```python
from build123d import *

# Parameters (mm, degrees)
SKETCH1_W           = 7
SKETCH1_H           = 65
SKETCH1_R           = 2.5
SKETCH1_H_2         = 33
BOSS_EXTRUDE1_DEPTH = 22.325
SKETCH2_R           = 17.825
CUT_EXTRUDE1_DEPTH  = 74.305222358
SKETCH3_R           = 6
CUT_EXTRUDE2_DEPTH  = 22.325


with BuildPart() as part:
    # Sketch1 → Boss-Extrude1 (new body)
    # profile 1 of 3: a face of its own
    with BuildSketch(Plane(origin=(0, 0, 0), x_dir=(1, 0, 0), z_dir=(0, 1, 0))):
        with Locations((22, 0)):
            Rectangle(SKETCH1_W, SKETCH1_H)
        with Locations(Location((22, -16.25, 0), (0, 0, 90))):
            Circle(SKETCH1_R, mode=Mode.SUBTRACT)
        with Locations(Location((22, 16.25, 0), (0, 0, 90))):
            Circle(SKETCH1_R, mode=Mode.SUBTRACT)
    # profile 2 of 3: a face of its own
    with BuildSketch(Plane(origin=(0, 0, 0), x_dir=(1, 0, 0), z_dir=(0, 1, 0))):
        with BuildLine():
            Line((-18.5, 32.5), (-18.5, -0.5))
            ThreePointArc((-18.5, -0.5), (-6.523379041, -14.840809158), (-0.42, -32.5))
            Line((-0.42, -32.5), (18.5, -32.5))
            Line((18.5, -32.5), (18.5, 32.5))
            Line((18.5, 32.5), (-18.5, 32.5))
        make_face()
    # profile 3 of 3: a face of its own
    with BuildSketch(Plane(origin=(0, 0, 0), x_dir=(1, 0, 0), z_dir=(0, 1, 0))):
        with Locations((-22, 16)):
            Rectangle(SKETCH1_W, SKETCH1_H_2)
        with Locations(Location((-22, 7.5, 0), (0, 0, 90))):
            Circle(SKETCH1_R, mode=Mode.SUBTRACT)
        with Locations(Location((-22, 24.5, 0), (0, 0, 90))):
            Circle(SKETCH1_R, mode=Mode.SUBTRACT)
    extrude(amount=BOSS_EXTRUDE1_DEPTH)

    # Sketch2 → Cut-Extrude1 (cut, through all)
    with BuildSketch(Plane(origin=(0, 0, -32.5), x_dir=(-1, 0, 0), z_dir=(0, 0, -1))):
        with Locations((0, 22.325)):
            Circle(SKETCH2_R)
        with BuildLine():
            Line((-17.825, 8.88345991), (-25.5, 8.88345991))
            Line((-25.5, 8.88345991), (-25.5, -2.88343075))
            Line((-25.5, -2.88343075), (25.5, -2.88343075))
            Line((25.5, -2.88343075), (25.5, 8.88345991))
            Line((25.5, 8.88345991), (17.825, 8.88345991))
            ThreePointArc((17.825, 8.88345991), (0, 0), (-17.825, 8.88345991))
        make_face()
    extrude(amount=-CUT_EXTRUDE1_DEPTH, mode=Mode.SUBTRACT)

    # Sketch3 → Cut-Extrude2 (cut)
    with BuildSketch(Plane.XZ.offset(-8.88345991)):
        with Locations((-22, -7.5)):
            Circle(SKETCH3_R)
        with Locations((22, -16.25)):
            Circle(SKETCH3_R)
        with Locations((22, 16.25)):
            Circle(SKETCH3_R)
        with Locations((-22, -24.5)):
            Circle(SKETCH3_R)
    extrude(amount=CUT_EXTRUDE2_DEPTH, mode=Mode.SUBTRACT)


with BuildPart() as body_2:
    # Mirror2: mirrored copy
    add(part.part.mirror(Plane(origin=(-25.5, 22.325, 0), x_dir=(0, 0, 1), z_dir=(-1, 0, 0))))


solid = body_2.part
```
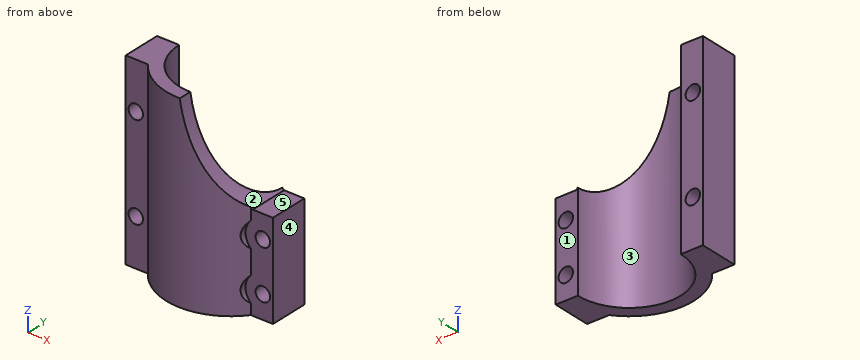
Model file for the job. Use its own axes, mm. Face numbers are marked on the shaded views. A direction names the side the tool comes from. Coordinates: 2 decimals unless noted, no trailing zeros. Order: outer loops, then holes, each group sorted by start corner. A loop starts at its lowest first (then second) coordinate and runs counter-clockwise, first axis right, second up. Notation, with made-up numbers: (31, 73) - (48, 73) arc R4 ccw to (48, 78) - close; hole circle Ø2 at (67, -38.5). An arc over 180 degrees is marked (long way). Return JSON: item names as keys, results as strings. Group by question number.
1) Mould opens along X. For the marked faces 1, 2 and 3 say: released by +X, released by -X, zero draft, split by the parting line, or undercut.
2) Saw through at A-A, the plane z = -7.5. Write the cut outline in (x, y) (3 decimals), plus the area to 3 significant figures.
3) Saw through at B-B, the plane y = 14. Write the cut outline in (x, z).
4) Saw through at C-C, the plane y = 20. Write the cut outline in (x, z), plus the area to 3 significant figures.
5) Flat gauge pins, fed straight in: P1, Ø8, axis at x = -39.5, z = 5.5, coming from the -Y side; P2, Ø10.5, axis at x = -28, z = -15, coming from the -Y side; P3, Ø5, axis at y = 10, z = 9.5, coming from the +X side; P4, Ø4.5, axis at x = -73, z = 16.25, coming from the -Y side. Where does each tip first touch, or does it go through?
6) Tool access for the marked faces 4 and 5: list every direction of +Z, -Z, +X, -X, +Y, -Y with a clear straight run to the whole face (end or side of a thin tool).
7) Saw through at D-D, the plane x = -34. Write the cut outline in (y, z), plus the area to 3 significant figures.
8) Probe line 1 (Z direction, x = -29, y = 17.75); line 2 (X direction, y = 17.75, z = -24.5); line 3 (X direction, y = 17.75, z = -6). List the from-to ranges inside material, lowest first. Write a range as from..to.
Values found:
{
 "1": {"face 1": "zero draft", "face 2": "released by +X", "face 3": "undercut"},
 "2": {"outline": "(-76.5, 8.883) - (-68.825, 8.883) arc R22.325 ccw to (-35, 6.756) - (-35, 8.883) - (-31.5, 8.883) - (-31.5, 22.325) - (-33.175, 22.325) arc R17.825 cw to (-68.825, 22.325) - (-76.5, 22.325) - close; (-26.5, 8.883) - (-25.5, 8.883) - (-25.5, 22.325) - (-26.5, 22.325) - close", "area": "338 mm²"},
 "3": {"outline": "(-76.5, -32.5) - (-66.76, -32.5) - (-66.76, 32.5) - (-76.5, 32.5) - close; (-35.24, -32.5) - (-25.5, -32.5) - (-25.5, 0.5) - (-32.5, 0.5) arc R51.75 cw to (-35.24, 2.95) - close; hole circle Ø5 at (-73, -16.25); hole circle Ø5 at (-73, 16.25); hole circle Ø5 at (-29, -24.5); hole circle Ø5 at (-29, -7.5)"},
 "4": {"outline": "(-76.5, -32.5) - (-68.67, -32.5) - (-68.67, 32.5) - (-76.5, 32.5) - close; (-33.33, -32.5) - (-25.5, -32.5) - (-25.5, 0.5) - (-32.5, 0.5) arc R51.75 cw to (-33.33, 1.2) - close; hole circle Ø5 at (-73, -16.25); hole circle Ø5 at (-73, 16.25); hole circle Ø5 at (-29, -24.5); hole circle Ø5 at (-29, -7.5)", "area": "689 mm²"},
 "5": {"P1": "stops at y = 1.3", "P2": "stops at y = 8.78", "P3": "stops at x = -39.24", "P4": "passes through"},
 "6": {"face 4": "+Z, -Z, +X, +Y, -Y", "face 5": "+Z, +X, +Y, -Y"},
 "7": {"outline": "(7.85, -32.5) - (16.96, -32.5) - (16.96, 1.8) - (7.85, 1.8) - (7.85, -4.18) - (8.88, -4.18) - (8.88, -10.82) - (7.85, -10.82) - (7.85, -21.18) - (8.88, -21.18) - (8.88, -27.82) - (7.85, -27.82) - close", "area": "299 mm²"},
 "8": {"line 1": "z = -32.5..-27, -22..-10, -5..0.5", "line 2": "x = -76.5..-68.23, -33.77..-31.5, -26.5..-25.5", "line 3": "x = -76.5..-68.23, -33.77..-31, -27..-25.5"}
}
